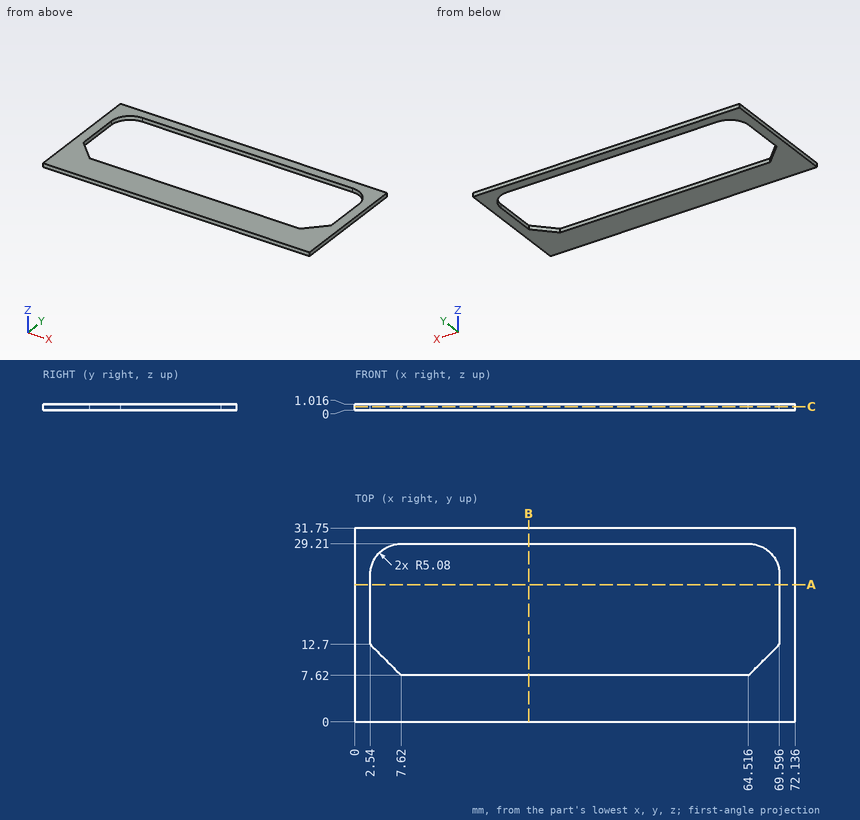
Input: dimensioned drawing with shaded views. Units: mm. Origin: part minimum x, y, z. Give positions to 0.01 mm unless a question says otherwise; leave off trailing zeros. Write each loop counter-clockwise with the first axis right and the second up, starting at its lowest first coordinate (ties: lowest second). Pieces come first, ordered by that corner, then holes.
Q1. Section A-A, the plane y = 22.5. Output: boundary loops of the cut face in (x, z).
Q2. Section B-B, the plane x = 28.5. Output: boundary loops of the cut face in (y, z), plus the area to 3 significant figures.
Q3. Section C-C, the plane z = 0.6. Output: boundary loops of the cut face in (x, y), plus the area to 3 significant figures.
Q4. Material intervals for probe 1 along Y at (x, z) = (52, 0.95); probe 2 along X at (y, z) = (19, 0.3); probe 3 along X at (y, z) = (10.5, 0.3), sorted ascending.
Filled in:
1. outline: (0, 0) - (2.54, 0) - (2.54, 1.02) - (0, 1.02) - close; (69.6, 0) - (72.14, 0) - (72.14, 1.02) - (69.6, 1.02) - close
2. outline: (0, 0) - (7.62, 0) - (7.62, 1.02) - (0, 1.02) - close; (29.21, 0) - (31.75, 0) - (31.75, 1.02) - (29.21, 1.02) - close
2. area: 10.3 mm2
3. outline: (0, 0) - (72.14, 0) - (72.14, 31.75) - (0, 31.75) - close; hole (2.54, 12.7) - (7.62, 7.62) - (64.52, 7.62) - (69.6, 12.7) - (69.6, 24.13) arc R5.08 ccw to (64.52, 29.21) - (7.62, 29.21) arc R5.08 ccw to (2.54, 24.13) - close
3. area: 879 mm2
4. probe 1: y = 0 to 7.62, 29.21 to 31.75
4. probe 2: x = 0 to 2.54, 69.6 to 72.14
4. probe 3: x = 0 to 4.74, 67.4 to 72.14
